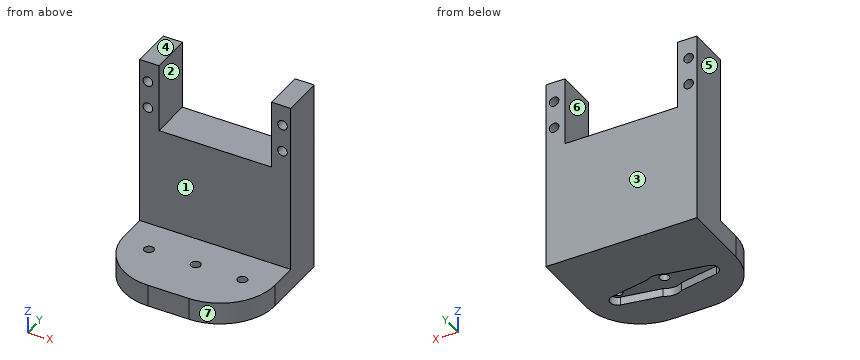
```python
from build123d import *

# Parameters (mm, degrees)
SKETCH1_W           = 55
SKETCH1_H           = 15
BOSS_EXTRUDE1_DEPTH = 70
SKETCH2_W           = 41
SKETCH2_H           = 15
CUT_EXTRUDE1_DEPTH  = 25
SKETCH3_R           = 1.75
CUT_EXTRUDE2_DEPTH  = 16
SKETCH4_W           = 55
SKETCH4_H           = 8
BOSS_EXTRUDE2_DEPTH = 30
FILLET1_R           = 20
CUT_EXTRUDE3_DEPTH  = 3
SKETCH6_R           = 1.75
CUT_EXTRUDE4_DEPTH  = 68


with BuildPart() as part:
    # Sketch1 → Boss-Extrude1 (new body)
    with BuildSketch(Plane.XY):
        Rectangle(SKETCH1_W, SKETCH1_H)
    extrude(amount=BOSS_EXTRUDE1_DEPTH)

    # Sketch2 → Cut-Extrude1 (cut)
    with BuildSketch(Plane.XY.offset(70)):
        Rectangle(SKETCH2_W, SKETCH2_H)
    extrude(amount=-CUT_EXTRUDE1_DEPTH, mode=Mode.SUBTRACT)

    # Sketch3 → Cut-Extrude2 (cut, through all)
    with BuildSketch(Plane(origin=(0, 7.5, 0), x_dir=(1, 0, 0), z_dir=(0, 1, 0))):
        with Locations((-24.5, -62.5)):
            Circle(SKETCH3_R)
        with Locations((24.5, -62.5)):
            Circle(SKETCH3_R)
        with Locations((-24.5, -52.5)):
            Circle(SKETCH3_R)
        with Locations((24.5, -52.5)):
            Circle(SKETCH3_R)
    extrude(amount=-CUT_EXTRUDE2_DEPTH, mode=Mode.SUBTRACT)

    # Sketch4 → Boss-Extrude2 (add)
    with BuildSketch(Plane(origin=(0, -7.5, 0), x_dir=(1, 0, 0), z_dir=(0, 1, 0))):
        with Locations((0, -4)):
            Rectangle(SKETCH4_W, SKETCH4_H)
    extrude(amount=-BOSS_EXTRUDE2_DEPTH)

    # Fillet1
    fillet1_edges = [part.edges().sort_by_distance(p)[0] for p in [
        (-27.5, -37.5, 4),
        (27.5, -37.5, 4),
    ]]
    fillet(fillet1_edges, radius=FILLET1_R)

    # Sketch5 → Cut-Extrude3 (cut)
    with BuildSketch(Plane(origin=(0, 0, 0), x_dir=(-1, 0, 0), z_dir=(0, 0, -1))):
        with BuildLine():
            Line((-17.477732777, -22.657399367), (-3.39236806, -25.189589478))
            ThreePointArc((-3.39236806, -25.189589478), (0, -26.2), (3.39236806, -25.189589478))
            Line((3.39236806, -25.189589478), (17.477732777, -22.657399367))
            ThreePointArc((17.477732777, -22.657399367), (19.7, -20), (17.477732777, -17.342600633))
            Line((17.477732777, -17.342600633), (3.39236806, -14.810410522))
            ThreePointArc((3.39236806, -14.810410522), (0, -13.8), (-3.39236806, -14.810410522))
            Line((-3.39236806, -14.810410522), (-17.477732777, -17.342600633))
            ThreePointArc((-17.477732777, -17.342600633), (-19.7, -20), (-17.477732777, -22.657399367))
        make_face()
    extrude(amount=-CUT_EXTRUDE3_DEPTH, mode=Mode.SUBTRACT)

    # Sketch6 → Cut-Extrude4 (cut, through all)
    with BuildSketch(Plane(origin=(0, 0, 3), x_dir=(-1, 0, 0), z_dir=(0, 0, -1))):
        with Locations((0, -20)):
            Circle(SKETCH6_R)
        with Locations((17, -20)):
            Circle(SKETCH6_R)
        with Locations((-17, -20)):
            Circle(SKETCH6_R)
    extrude(amount=-CUT_EXTRUDE4_DEPTH, mode=Mode.SUBTRACT)


solid = part.part
```
The listing builds one solid part. Answer for the finished solid, in the listing's coordinates (mm). Face numbers are marked on the shaded views. A direction names the side the tool comes from. Round coordinates to 2 decimals unless told otherwise and drop trailing zeros. Loops run counter-clockwise (first coordinate to the right, second up) from the corner with the lowest first, then second, coordinate; pieces in that order, holes last. Notation, with made-up numbers: (-35.75, -21) - (2.25, -21) arc R10 cw to (2.25, -14) - close; hole circle Ø5 at (24, 39). An arc over 180 degrees is marked (long way). Return JSON: item names as keys, results as strings. Group by question number.
1. The part is cut by section A-A on x = 0. Determine the outline of the cut face in (y, z).
2. The part is cut by section C-C on z = 52.5. Determine the outline of the cut face in (x, y).
3. The part is cut by section D-D on x = 24. Determine the outline of the cut face in (y, z).
4. The part is cut by section B-B on y = -2. Determine the outline of the cut face in (x, z).
5. Each of these flat-tipped pins is pushed along its axis until it touches: P1, Ø5.5, axis at x = 17, y = -20, coming from the +Z side; P2, Ø7.5, axis at x = 8, y = -0.5, coming from the +Z side; P3, Ø4.5, axis at x = -17, y = -20, coming from the -Z side. Where does it stop, or does it pass through?
6. Consider probe 1 along X at (y, z) = (3.5, 52.5); probe 2 along Z at (x, y) = (-24.5, 4.5); probe 3 along X at (y, z) = (-20.5, 4). Determine where each line is inside the solid, lowest interval first.
7. Which of the six approach directions +Z, -Z, +X, -X, +Y, -Y give full straight-line access (tool end or side, diameter ignored) to the marked faces 1, 2 and 3?
8. The mould has two halves that part along X. Classify the marked faces 4, 5, 6 and 7: pulls with the +X half, pulls with the -X half, needs draft (parallel to the pull), parting line crosses it, or undercut.
Resolved:
{
 "1": {"outline": "(-37.5, 0) - (-26.2, 0) - (-26.2, 3) - (-21.75, 3) - (-21.75, 8) - (-37.5, 8) - close; (-18.25, 3) - (-13.8, 3) - (-13.8, 0) - (7.5, 0) - (7.5, 45) - (-7.5, 45) - (-7.5, 8) - (-18.25, 8) - close"},
 "2": {"outline": "(-27.5, -7.5) - (-26.25, -7.5) - (-26.25, 7.5) - (-27.5, 7.5) - close; (-22.75, -7.5) - (-20.5, -7.5) - (-20.5, 7.5) - (-22.75, 7.5) - close; (20.5, -7.5) - (22.75, -7.5) - (22.75, 7.5) - (20.5, 7.5) - close; (26.25, -7.5) - (27.5, -7.5) - (27.5, 7.5) - (26.25, 7.5) - close"},
 "3": {"outline": "(-28.8, 0) - (7.5, 0) - (7.5, 50.82) - (-7.5, 50.82) - (-7.5, 8) - (-28.8, 8) - close; (-7.5, 54.18) - (7.5, 54.18) - (7.5, 60.82) - (-7.5, 60.82) - close; (-7.5, 64.18) - (7.5, 64.18) - (7.5, 70) - (-7.5, 70) - close"},
 "4": {"outline": "(-27.5, 0) - (27.5, 0) - (27.5, 70) - (20.5, 70) - (20.5, 45) - (-20.5, 45) - (-20.5, 70) - (-27.5, 70) - close; hole circle Ø3.5 at (-24.5, 52.5); hole circle Ø3.5 at (-24.5, 62.5); hole circle Ø3.5 at (24.5, 52.5); hole circle Ø3.5 at (24.5, 62.5)"},
 "5": {"P1": "stops at z = 8", "P2": "stops at z = 45", "P3": "stops at z = 3"},
 "6": {"probe 1": "x = -27.5 to -26.25, -22.75 to -20.5, 20.5 to 22.75, 26.25 to 27.5", "probe 2": "z = 0 to 50.75, 54.25 to 60.75, 64.25 to 70", "probe 3": "x = -27.27 to -18.68, -15.32 to -1.68, 1.68 to 15.32, 18.68 to 27.27"},
 "7": {"face 1": "+Z, +X, -X, -Y", "face 2": "+Z, +Y, -Y", "face 3": "+Z, -Z, +X, -X, +Y"},
 "8": {"face 4": "needs draft", "face 5": "pulls with the -X half", "face 6": "undercut", "face 7": "pulls with the +X half"}
}
